```python
from build123d import *

# Parameters (mm, degrees)
F1_DEPTH = 25.4
F2_R     = 50.79999
F3_R     = 25.4
F4_DEPTH = 79.248


# Not quite as in the source:
# - a fillet or chamfer is up to 0.001 mm smaller than in the source, because OpenCascade refuses the exact size


with BuildPart() as f1:
    # F0 (on Front) → F1 (new body)
    with BuildSketch(Plane.XZ):
        with BuildLine():
            ThreePointArc((0, -50.8), (35.9210244843, -35.9210244843), (50.8, 0))
            ThreePointArc((50.8, 0), (35.9210244843, 35.9210244843), (0, 50.8))
            Line((0, 50.8), (0, -50.8))
        make_face()
        with BuildLine():
            ThreePointArc((0, 50.8), (35.9210244843, 35.9210244843), (50.8, 0))
            ThreePointArc((50.8, 0), (35.9210244843, -35.9210244843), (0, -50.8))
            Line((0, -50.8), (127, -50.8))
            Line((127, -50.8), (127, 50.8))
            Line((127, 50.8), (0, 50.8))
        make_face()
        with BuildLine():
            Line((0, -50.8), (0, 50.8))
            ThreePointArc((0, 50.8), (-50.8, 0), (0, -50.8))
        make_face()
    extrude(amount=F1_DEPTH)

    # F2 (radius 50.8 in the source; OpenCascade refuses exactly that, so slightly less here)
    f2_edges = [f1.edges().sort_by_distance(p)[0] for p in [
        (127, -12.7, 50.8),
        (127, -12.7, -50.8),
    ]]
    fillet(f2_edges, radius=F2_R)

    # F3 (on Front) → F4 (cut)
    with BuildSketch(Plane.XZ):
        Circle(F3_R)
    f4 = extrude(amount=F4_DEPTH, mode=Mode.SUBTRACT)

    # F7: F4 across plane
    add(f4.mirror(Plane.YZ.offset(38.1)), mode=Mode.SUBTRACT)


solid = f1.part
```
Can you work these out from the model? Positions are in its coordinate system, mm. Coordinates: 2 decimals unless noted, no trailing zeros. Loops run counter-clockwise (first coordinate to the right, second up) from the corner with the lowest first, then second, coordinate; pieces in that order, holes last. Notation, with made-up numbers: (4.5, 87.5) -> (34.5, 87.5) arc R16 cw to (34.5, 109.5) -> close; hole circle Ø10 at (-8, 14.5). An arc over 180 degrees is marked (long way). Put each result on its own line as item: value. Start each with the question number.
Q1. I want a section at B-B (x = 89). Write out the boundary of the cut face in (y, z), plus the area to 3 significant figures.
Q2. If I drill on line 1 (X direction, y = -21.5, z = 3.5); line 2 (Z direction, x = -0.5, y = -13.5); line 3 (X direction, y = -14.25, z = 6), over which ranges is the centre line in solid material (lowest first)? Write a range as [from, to].
Q3. I'm going to push flat-ended pins straight in: P1, Ø6, axis at y = -11, z = -30.5, coming from the +X side; P2, Ø12, axis at x = -7, y = -19.5, coming from the +Z side; P3, Ø1, axis at y = -11.5, z = -12, coming from the +X side. Where does each tip first touch, or does it pass through?
Q4. I want a section at C-C (y = -16.75). Count the separate pieces of the cut face and the enclosed holes in it, plus the area to 3 significant figures.
Q5. I want a section at D-D (z = -4). Write out the boundary of the cut face in (x, y), plus the area to 3 significant figures.
Q6. I want a section at A-A (z = 14). Write out the boundary of the cut face in (x, y).
Q7. Thinking about a two-plate mould opening in X: for faces 1 (the face through (-5.506, -12.522, -24.796)), 2 (the face through (39, -13, 50.8)), 3 (the face through (112.514, -12.878, 35.524)), 4 (the face through (-50.788, -12.522, 1.117)), which applies, pulls with the +X half, pulls with the -X half, needs draft (parallel to the pull), parting line crosses it, or undercut?
Taken from the geometry:
1. outline: (-25.4, -49.16) -> (0, -49.16) -> (0, -21.94) -> (-25.4, -21.94) -> close; (-25.4, 21.94) -> (0, 21.94) -> (0, 49.16) -> (-25.4, 49.16) -> close
1. area: 1,380 mm2
2. line 1: x = [-50.68, -25.16], [25.16, 51.04], [101.36, 126.88]
2. line 2: z = [-50.8, -25.4], [25.4, 50.8]
2. line 3: x = [-50.44, -24.68], [24.68, 51.52], [100.88, 126.64]
3. P1: stops at x = 118.91
3. P2: stops at z = 50.79
3. P3: stops at x = 125.68
4. separate pieces: 1
4. enclosed holes: 2
4. area: 11,800 mm2
5. outline: (-50.64, -25.4) -> (-25.08, -25.4) -> (-25.08, 0) -> (-50.64, 0) -> close; (25.08, -25.4) -> (51.12, -25.4) -> (51.12, 0) -> (25.08, 0) -> close; (101.28, -25.4) -> (126.84, -25.4) -> (126.84, 0) -> (101.28, 0) -> close
5. area: 1,960 mm2
6. outline: (-48.83, -25.4) -> (-21.19, -25.4) -> (-21.19, 0) -> (-48.83, 0) -> close; (21.19, -25.4) -> (55.01, -25.4) -> (55.01, 0) -> (21.19, 0) -> close; (97.39, -25.4) -> (125.03, -25.4) -> (125.03, 0) -> (97.39, 0) -> close
7. face 1: undercut
7. face 2: needs draft
7. face 3: pulls with the +X half
7. face 4: pulls with the -X half
